Can you work these out from the model? Positions are in its coordinate system, mm. Give positions to 0.01 mm unless a question says otherwise; leave off trailing zeros. Order: outer loops, then holes, each group sorted by start corner. A loop starts at its lowest first (then second) coordinate and runs counter-clockwise, first axis right, second up. Notation, with made-up numbers: (2, 20) - (24, 20) arc R22 ccw to (24, 45) - close; hole circle Ø7 at (51, 4.5). An arc over 180 degrees is marked (long way). Return JSON: item names as keys, results as strings.
Autodesk Inventor part; units mm, degrees
ref_plane "MSC_PF1" through (0, 0, 0) normal (1, 0, 0) x (0, 1, 0)
ref_plane "MSC_PT1" through (0, 0, 0) normal (0, 0, -1) x (-1, 0, 0)
ref_plane "YZ Plane" through (0, 0, 0) normal (1, 0, 0) x (0, 1, 0)
sketch "Esquisse1" plane through (0, 0, 0) normal (0, 1, 0) x (-1, 0, 0)
  point P0 (0, 0)
sketch "Esquisse2" plane through (0, 0, 0) normal (0, 0, 1) x (1, 0, 0)
  point P0 (0, 0)
sketch "Esquisse3" plane through (0, 0, 0) normal (0, 0, 1) x (1, 0, 0)
  point P0 (0, 0)
sketch "Esquisse4" plane through (0, 0, 0) normal (0, 1, 0) x (-1, 0, 0)
  line L0 (-2.75, 0) -> (0, 0)
  line L1 (-2.75, -0.4) -> (-2.75, 0)
  line L2 (-1.5, -1.65) -> (-2.75, -0.4)
  line L3 (-1.5, -1.9) -> (-1.5, -1.65)
  line L4 (-1.25, -2.15) -> (-1.5, -1.9)
  line L5 (-1.5, -2.4) -> (-1.25, -2.15)
  line L6 (-1.5, -8) -> (-1.5, -2.4)
  line L7 (0, 0) -> (0, -8)
  line L8 (0, 3.3392) -> (0, -10.7) construction
  line L9 (0, 3.3392) -> (0, -10.7)
  line L10 (0, -13.5078) -> (0, 6.1471)
  line L11 (-1.5, -8) -> (0, -8)
  line L12 (0.55, 0) -> (-3.3, 0)
  dimension "d3" = 2.75
  dimension "d5" = 0.25
  dimension "d7" = 0.25
  dimension "d9" = 0.25
  dimension "d11" = 1.65
  dimension "d13" = 135
  dimension "d17" = 1.25
  dimension "d19" = 0
  dimension "d51" = 1.5
  dimension "d52" = 8
revolve "Révolution1" add sketch "Esquisse4" angle 360 about axis through (0, 0, 3.3392) along (0, 0, -1)
sketch "Esquisse5" plane through (0, 0, 0) normal (0, 1, 0) x (-1, 0, 0)
  line L0 (-1.6, 0) -> (0, 0)
  line L1 (-0.2667, -1.5) -> (-1.6, 0)
  line L2 (0, -1.5) -> (-0.2667, -1.5)
  line L3 (0, 0) -> (0, -1.5)
  line L4 (-1.5, -1.65) -> (1.5, -1.65) construction
  line L5 (-2.75, 0) -> (2.75, 0)
  line L6 (0, -1.98) -> (0, 0.33)
  dimension "d22" = 1.6
  dimension "d24" = 0.2667
  dimension "d26" = 1.5
extrude "Extrusion1" cut sketch "Esquisse5" along normal mid plane 0.5333
pattern_circular "RéseauPolaire1" count 4 over 360 about axis through (0, 0, 0) along (0, 0, 1) of "Extrusion1"
sketch "Esquisse7" plane through (0, 0, 0) normal (0, 1, 0) x (-1, 0, 0)
  line L0 (0, -0.825) -> (-2, 0)
  line L1 (0, 0) -> (0, -0.825)
  line L2 (-2, 0) -> (0, 0)
  line L3 (-1.5, -1.65) -> (1.5, -1.65) construction
  line L4 (0, -1.98) -> (0, 0.33)
  line L5 (-2.75, 0) -> (2.75, 0)
  dimension "d33" = 2
  dimension "d35" = 0.825
extrude "Extrusion2" cut sketch "Esquisse7" along normal mid plane 0.5333
pattern_circular "RéseauPolaire2" count 4 over 360 about axis through (0, 0, 0) along (0, 0, 1) of "Extrusion2"
fillet "Congé1" radius 0.5 1 edges at (-1.5, 0, -1.65)
thread "Filetage1"
ref_plane "MSC_PF1" through (0, 0, 0) normal (1, 0, 0) x (0, 1, 0)
ref_plane "MSC_PT1" through (0, 0, 0) normal (0, 0, -1) x (-1, 0, 0)
equation "\"d3\" = 0.5 * Dh"
equation "\"d5\" = msp_x"
equation "\"d7\" = ParA"
equation "\"d9\" = msp_x"
equation "\"d11\" = ParK"
equation "\"d17\" = 0.5 * msp_mdtds"
equation "\"d51\" = 0.5 * NND"
equation "\"d52\" = NLG"
equation "\"d22\" = 0.5 * M"
equation "\"d24\" = 0.0833333 * M"
equation "\"d26\" = 0.909091 * ParK"
equation "\"d27\" = 0.166667 * M"
equation "\"d33\" = 0.625 * M"
equation "\"d35\" = 0.5 * ParK"
equation "\"d36\" = 0.166667 * M"
equation "\"d41\" = 2 * msp_x"
equation "\"PTC\" = 0.5"
equation "\"NLG\" = 8"
equation "\"ParK\" = 1.65"
equation "\"NND\" = 3"
equation "\"M\" = 3.2"
equation "\"msp_mdtds\" = NND - PTC"
equation "\"Dh\" = 5.5"
equation "\"msp_x\" = 0.5 * PTC"
equation "\"ParA\" = 0.5 * PTC"
equation "\"r\" = 0.8"
equation "\"THREADDIA\" = NND"
equation "\"TEMPLATE\" = 1.2345"
properties part number "NF EN ISO 7046-2 H - M3x8 - 8.8 - H1" material "Acier inoxydable 440C"
1. Thinking about a two-plate mould opening in Y: for faces 1 (the face through (0, 0.8, -0.9)), 2 (the face through (-1.5, 0.07, -5.16)), 3 (the face through (0, 0, -8)), which applies, +Y half, -Y half, draft (parallel to the pull), parting line (faces both ways), or undercut?
Checks:
{"face 1": "undercut", "face 2": "parting line", "face 3": "draft"}
2. If I drill on L1, parallel to Y at x = 0.7, z = -0.25; L2, parallel to X at y = 0, z = -6.75; L3, parallel to X at y = -0.65, z = -1, over which ranges is the centre line in solid material (lowest first)? Write a range as [from, to].
Checks:
{"L1": "[-2.66, -0.27], [0.27, 2.66]", "L2": "[-1.5, 1.5]", "L3": "[-2.05, -0.27], [0.27, 2.05]"}
3. For pin 1 Ø1 at (y, z) = (-1.5, -7) entering from -X; pin 2 Ø2 at (x, z) = (-1, -3.5) entering from +Y; pin 3 Ø2 at (x, z) = (-1.5, -2) entering from +Y, each with a flat end and sliding along its axis, tell me the tip position at first contact or that it passes through.
Checks:
{"pin 1": "x = -1.12", "pin 2": "y = 1.5", "pin 3": "y = 1.75"}
4. Suppose I cut it at A-A (z = -2). List the corners of the cut face in (x, y) for me.
Checks:
{"outline": "circle Ø2.8 at (0, 0)"}
5. Suppose I cut it at B-B (z = -6.25). List the corners of the cut face in (x, y) for me.
Checks:
{"outline": "circle Ø3 at (0, 0)"}
